For this review, take the finished solid that the model builds, in its own axes (mm). Face numbers are marked on the shaded views. A direction names the side the tool comes from. Round coordinates to 2 decimals unless told otherwise and drop trailing zeros. Order: outer loops, then holes, each group sorted by start corner. A loop starts at its lowest first (then second) coordinate and runs counter-clockwise, first axis right, second up. Notation, with made-up numbers: (-21.75, 14.25) - (1.25, 14.25) arc R21 ccw to (1.25, 23.25) - close; hole circle Ø2 at (1.5, 2). An arc over 180 degrees is marked (long way). One line per item, written item: value.
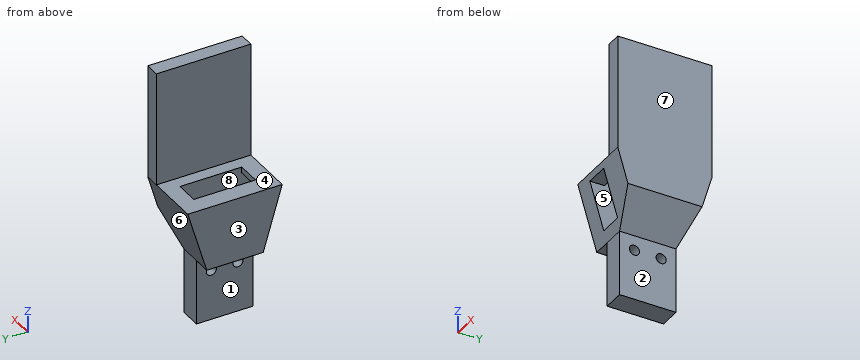
Autodesk Inventor part; units mm, degrees
ref_plane "YZ Plane" through (0, 0, 0) normal (1, 0, 0) x (0, 1, 0)
ref_plane "XZ Plane" through (0, 0, 0) normal (0, 1, 0) x (-1, 0, 0)
ref_plane "XY Plane" through (0, 0, 0) normal (0, 0, 1) x (1, 0, 0)
sketch "Sketch1" plane through (0, 0, 0) normal (1, 0, 0) x (0, 1, 0)
  line L0 (0, 0) -> (19, 0)
  line L1 (19, 0) -> (19, 22)
  line L2 (19, 22) -> (0, 22)
  line L3 (0, 22) -> (0, 0)
  line L4 (19, 22) -> (14, 22)
  line L5 (14, 22) -> (14, 17)
  line L6 (14, 17) -> (19, 17)
  line L7 (19, 17) -> (19, 22)
  line L8 (0, 22) -> (5, 22)
  line L9 (5, 22) -> (5, 17)
  line L10 (5, 17) -> (0, 17)
  line L11 (0, 17) -> (0, 22)
  circle A0 centre (14, 17) radius 1.7
  circle A1 centre (5, 17) radius 1.7
  dimension "d0" = 19
  dimension "d1" = 22
  dimension "d2" = 5
  dimension "d3" = 5
  dimension "d4" = 5
  dimension "d5" = 5
  dimension "d6" = 3.4
  dimension "d7" = 3.4
extrude "Extrusion1" add sketch "Sketch1" along normal blind 17.2 contours L3 L10 A1 L9 L2 L5 A0 L6 L1 L0 | L3 L2 L9 A1 L10 | L6 A0 L5 L2 L1
sketch "Sketch2" plane through (0, 19, 22) normal (0, 1, 0) x (1, 0, 0)
  line L0 (0, 0) -> (17.2, 0)
  line L1 (17.2, 0) -> (-6, 0)
  line L2 (-6, 0) -> (-6, -60)
  line L3 (-6, -60) -> (17.2, -60)
  line L4 (17.2, -60) -> (17.2, 0)
  point P0 (0, 22)
  dimension "d10" = 23.2
  dimension "d11" = 60
extrude "Extrusion2" add sketch "Sketch2" against normal blind 19
sketch "Sketch3" plane through (-6, 19, 22) normal (-1, 0, 0) x (0, 0, 1)
  line L0 (-22, 0) -> (60, 0)
  line L1 (-22, -19) -> (60, -19)
  line L2 (60, 0) -> (21.5, 0)
  line L3 (21.5, 0) -> (21.5, -19)
  line L4 (21.5, -19) -> (60, -19)
  line L5 (60, -19) -> (60, 0)
  point P0 (-10, 0)
  point P1 (-10, -19)
  dimension "d23" = 38.5
extrude "Extrusion3" cut sketch "Sketch3" against normal blind 18.2
sketch "Sketch4" plane through (17.2, 0, 0) normal (1, 0, 0) x (0, 0, -1)
  line L0 (0, 0) -> (0, 19)
  line L1 (0, 19) -> (-82, 19)
  line L2 (0, 0) -> (-22, 0)
  line L3 (-22, 0) -> (-22, 19)
  line L4 (-22, 19) -> (0, 19)
  line L5 (0, 19) -> (0, 0)
  dimension "d26" = 22
extrude "Extrusion4" cut sketch "Sketch4" against normal blind 10
sketch "Sketch5" plane through (17.2, 0, 0) normal (1, 0, 0) x (0, 0, -1)
  line L0 (-22, 0) -> (-22, 19)
  line L1 (-22, 9.5) -> (-22, 25.4)
  line L2 (-43.5, 0) -> (-43.5, 19)
  line L3 (-22, 25.4) -> (-43.5, 25.4)
  line L4 (-43.5, 25.4) -> (-43.5, 19)
  line L5 (-43.5, 19) -> (-22, 19)
  line L6 (-22, 19) -> (-22, 25.4)
  line L7 (0, 19) -> (-22, 19)
  line L8 (-43.5, 25.4) -> (-22, 19)
  line L9 (-22, 9.5) -> (-27.2776, 9.5)
  line L10 (-22, 19) -> (-22, 0)
  line L11 (-22, 9.5) -> (-22, -6.4)
  line L12 (-43.5, 19) -> (-43.5, 0)
  line L13 (-22, -6.4) -> (-43.5, -6.4)
  line L14 (-43.5, -6.4) -> (-43.5, 0)
  line L15 (-43.5, 0) -> (-22, 0)
  line L16 (-22, 0) -> (-22, -6.4)
  line L17 (0, 0) -> (-22, 0)
  line L18 (-43.5, -6.4) -> (-22, 0)
  point P0 (0, 0)
  dimension "d29" = 15.9
extrude "Extrusion5" add sketch "Sketch5" against normal blind 23.2 contours L18 L14 L15 | L5 L4 L8
sketch "Sketch6" plane through (17.2, 0, 0) normal (1, 0, 0) x (0, 0, -1)
  line L0 (-82, 19) -> (-82, 0)
  line L1 (-43.5, -6.4) -> (-43.5, 25.4)
  line L2 (-82, 0) -> (-43.5, 0)
  line L3 (-43.5, 0) -> (-43.5, -6.4)
  line L4 (-43.5, -6.4) -> (-82, -6.4)
  line L5 (-82, -6.4) -> (-82, 0)
  line L6 (-43.5, 19) -> (-82, 19)
  line L7 (-43.5, 25.4) -> (-22, 19)
  line L8 (-82, 19) -> (-43.5, 19)
  line L9 (-43.5, 19) -> (-43.5, 25.4)
  line L10 (-43.5, 25.4) -> (-82, 25.4)
  line L11 (-82, 25.4) -> (-82, 19)
  point P0 (0, 0)
extrude "Extrusion6" add sketch "Sketch6" against normal blind 5 contours L11 L10 L1 L6 | L2 L1 L4 L5
chamfer "Chamfer4" distance 10 angle 45 1 edges at (17.2, 9.5, 22)
ref_plane "Work Plane1" through (8, -6.4, 43.5) normal (-1, 0, 0) x (0, 0, 1)
sketch "Sketch11" plane through (8, -6.4, 43.5) normal (-1, 0, 0) x (0, 0, 1)
  line L0 (38.5, 31.8) -> (0, 31.8)
  line L1 (38.5, 0) -> (0, 0)
  line L2 (0, 31.8) -> (0, 0)
  line L3 (0, 0) -> (0, 31.8)
  line L4 (0, 15.9) -> (0, 5.5)
  line L5 (0, 5.5) -> (0, 26.3)
  line L6 (0, 26.3) -> (-14, 26.3)
  line L7 (-14, 26.3) -> (-19.2094, -3.2442)
  line L8 (0, 5.5) -> (-2, 5.5)
  line L9 (-2, 5.5) -> (-2, -4.5)
  line L10 (-19.2094, -3.2442) -> (-2, -4.5)
  point P0 (-43.5, 6.4)
  dimension "d61" = 10.4
  dimension "d62" = 20.8
  dimension "d63" = 14
  dimension "d64" = 30
  dimension "d65" = 100
  dimension "d66" = 2
  dimension "d67" = 10
  dimension "d68" = 90
extrude "Extrusion10" cut sketch "Sketch11" along normal blind 8
sketch "Sketch12" plane through (12.2, 19, 22) normal (-1, 0, 0) x (0, 0, 1)
  point P0 (-22, -19)
properties part number "Finger"
Item 1: Wall thickness on line 1 (Y direction, x = 4, z = 17); line 2 (X direction, y = 9, z = 77.5); line 3 (Y direction, x = 3, z = 4.5): over which ranges is each line inside the solid? List them lowest first.
Returned:
line 1: 0 to 3.3, 6.7 to 12.3, 15.7 to 19
line 2: 12.2 to 17.2
line 3: 0 to 19
Item 2: Take a section at B-B (x = 4). Write out the cut boundary in (y, z).
Returned:
outline: (-6.4, 43.5) - (-5.8, 41.5) - (-0.9, 41.5) - (-0.9, 43.5) - close; (-1.13, 25.79) - (0, 22) - (0, 0) - (19, 0) - (19, 22) - (25.4, 43.5) - (19.9, 43.5) - (19.9, 29.5) - close; hole circle Ø3.4 at (5, 17); hole circle Ø3.4 at (14, 17)
Item 3: The part is to be moulded in two halves that separate along X. For the marked faces 5, 6, 7 and 8, say which applies: +X half, -X half, draft (parallel to the pull), parting line (faces both ways), or undercut.
Returned:
face 5: undercut
face 6: draft
face 7: +X half
face 8: undercut
Item 4: Take a section at A-A (z = 17). Write out the cut boundary in (x, y).
Returned:
outline: (0, 0) - (7.2, 0) - (7.2, 3.3) - (0, 3.3) - close; (0, 6.7) - (7.2, 6.7) - (7.2, 12.3) - (0, 12.3) - close; (0, 15.7) - (7.2, 15.7) - (7.2, 19) - (0, 19) - close
Item 5: Take a section at D-D (z = 40.5). Write out the cut boundary in (x, y), plus the area to 3 significant figures.
Returned:
outline: (-6, -5.51) - (0, -5.51) - (0, 19.9) - (8, 19.9) - (8, -5.51) - (17.2, -5.51) - (17.2, 24.51) - (-6, 24.51) - close
area: 493 mm^2
Item 6: For P1, Ø10, axis at y = 3, z = 12, coming from the -X side; P2, Ø15, axis at y = 7.5, z = 13, coming from the +X side; P3, Ø10, axis at y = 13.5, z = 19, coming from the -X side; P4, Ø1.8, axis at x = -2.5, y = 13.5, coming from the -Z side, all flat-tipped, find the tip position at first contact; note any pin that passes through.
Returned:
P1: x = 0
P2: x = 7.2
P3: x = -6
P4: z = 22
Item 7: Machinability: for the marked faces 1, 2, 3 and 4, which of the approach directions +Z, -Z, +X, -X, +Y, -Y give a long, thin tool a straight path to every point of the face, cutting with its end or side? Answer none if there is none.
Returned:
face 1: -Z, -X, +Y, -Y
face 2: -Z, +X, +Y, -Y
face 3: +Z, -Z, -X, +Y, -Y
face 4: +Z, -X, +Y, -Y
